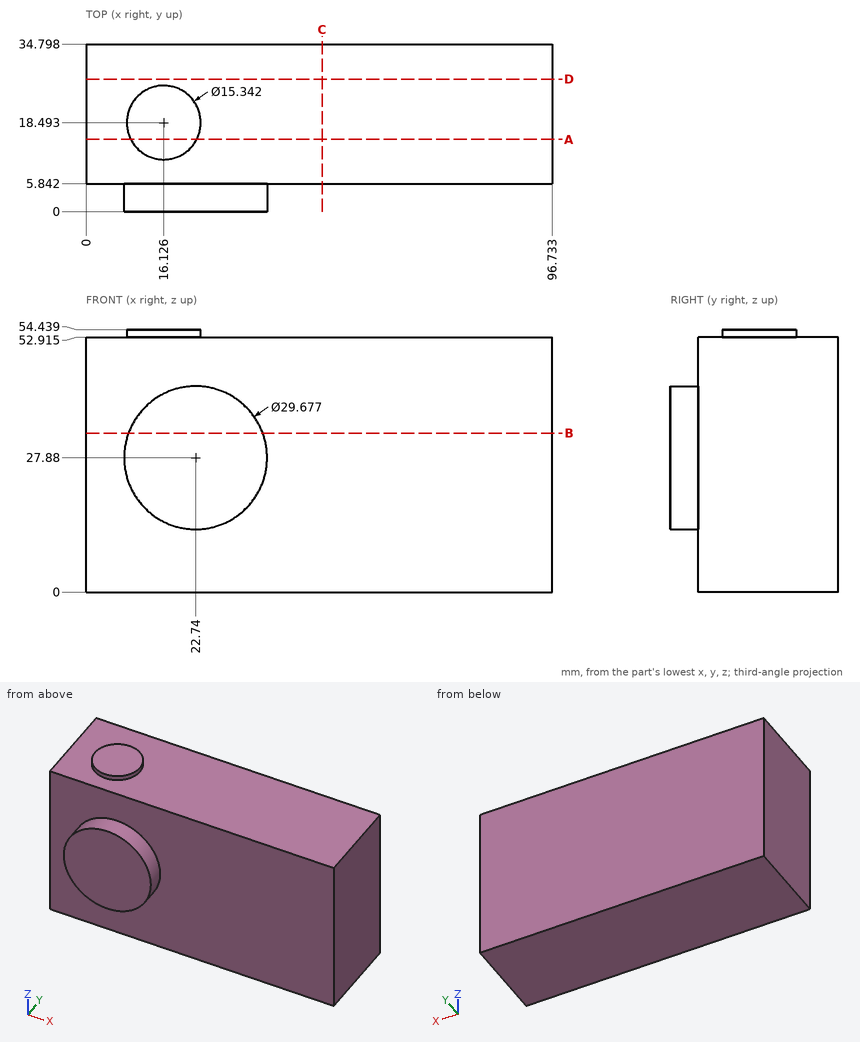
The drawing under review shows one solid part. Ordinate dimensions are in mm from its lowest x, y, z. Give positions to 0.01 mm unless a question says otherwise; leave off trailing zeros. Write each loop counter-clockwise with the first axis right and the second up, starting at its lowest first coordinate (ties: lowest second). Pieces come first, ordered by that corner, then holes. Notation, with made-up numbers: (27.25, -6.75) -> (61.25, -6.75) arc R33 ccw to (61.25, 29.25) -> close; hole circle Ø1 at (-17, 82.25). An arc over 180 degrees is marked (long way). Answer in a Markdown table with one row per item.
(1) Consider section D-D (y = 27.5). State the section outline as (x, z) points (1 decimal), then the cut area to 3 significant figures.
Results:
| item | result |
|---|---|
| outline | (0, 0) -> (96.7, 0) -> (96.7, 52.9) -> (0, 52.9) -> close |
| area | 5,120 mm2 |
(2) Consider section B-B (z = 33). State the section outline as (x, y) points.
Results:
| item | result |
|---|---|
| outline | (0, 5.84) -> (8.81, 5.84) -> (8.81, 0) -> (36.67, 0) -> (36.67, 5.84) -> (96.73, 5.84) -> (96.73, 34.8) -> (0, 34.8) -> close |
(3) Consider section A-A (y = 15). State the section outline as (x, z) points (1 decimal).
Results:
| item | result |
|---|---|
| outline | (0, 0) -> (96.7, 0) -> (96.7, 52.9) -> (23, 52.9) -> (23, 54.4) -> (9.3, 54.4) -> (9.3, 52.9) -> (0, 52.9) -> close |
(4) To check wall thickness, follow probe 1 along Z at (x, y) = (87.5, 32) (1 decimal); probe 2 along Y at (x, z) = (36, 45.5); probe 3 along Z at (x, y) = (9.5, 5) (1 decimal). State the ranges of each line that lie inside material, in increasing order.
Results:
| item | result |
|---|---|
| probe 1 | 0 to 52.9 |
| probe 2 | 5.84 to 34.8 |
| probe 3 | 21.2 to 34.6 |
(5) Consider section C-C (x = 49). State the section outline as (y, z) points (1 decimal), then the cut area to 3 significant figures.
Results:
| item | result |
|---|---|
| outline | (5.8, 0) -> (34.8, 0) -> (34.8, 52.9) -> (5.8, 52.9) -> close |
| area | 1,530 mm2 |
(6) Clearance check with flat-ended pins moving along their axes: pin 1 (6 mm diameter, centred on x = 22.5, y = 28.5, fed in from +Z) (1 decimal); pin 2 (5 mm diameter, centred on x = 42.5, z = 38.5, fed in from -Y). State where each tip first meets the part, or that it passes through.
Results:
| item | result |
|---|---|
| pin 1 | z = 52.9 |
| pin 2 | y = 5.84 |
